from build123d import *

# Parameters (mm, degrees)
SKETCH1_W           = 110.344434204
SKETCH1_H           = 22.05
BOSS_EXTRUDE1_DEPTH = 3
SKETCH3_W           = 10.2
SKETCH3_H           = 3.2
SKETCH3_W_2         = 3.2
SKETCH3_H_2         = 10.372217102
CUT_EXTRUDE1_DEPTH  = 4


with BuildPart() as part:
    # Sketch1 → Boss-Extrude1 (new body)
    with BuildSketch(Plane(origin=(0, 0, 0), x_dir=(1, 0, 0), z_dir=(0, 1, 0))):
        with Locations((0, -55.817990858)):
            Rectangle(SKETCH1_W, SKETCH1_H)
    extrude(amount=-BOSS_EXTRUDE1_DEPTH)

    # Sketch3 → Cut-Extrude1 (cut, through all)
    with BuildSketch(Plane(origin=(0, 0, 0), x_dir=(1, 0, 0), z_dir=(0, 1, 0))):
        with Locations((-40, -46.292990858)):
            Rectangle(SKETCH3_W, SKETCH3_H)
        with Locations((-53.672217102, -61.756882307)):
            Rectangle(SKETCH3_W_2, SKETCH3_H_2)
        with Locations((53.672217102, -65.342990858)):
            Rectangle(SKETCH3_W_2, SKETCH3_H)
        with Locations((-40, -65.342990858)):
            Rectangle(SKETCH3_W, SKETCH3_H)
        with Locations((-20, -46.292990858)):
            Rectangle(SKETCH3_W, SKETCH3_H)
        with Locations((-20, -65.342990858)):
            Rectangle(SKETCH3_W, SKETCH3_H)
        with Locations((0, -46.292990858)):
            Rectangle(SKETCH3_W, SKETCH3_H)
        with Locations((0, -65.342990858)):
            Rectangle(SKETCH3_W, SKETCH3_H)
        with Locations((20, -46.292990858)):
            Rectangle(SKETCH3_W, SKETCH3_H)
        with Locations((20, -65.342990858)):
            Rectangle(SKETCH3_W, SKETCH3_H)
        with Locations((40, -46.292990858)):
            Rectangle(SKETCH3_W, SKETCH3_H)
        with Locations((40, -65.342990858)):
            Rectangle(SKETCH3_W, SKETCH3_H)
        with Locations((-40, -57.242990858)):
            Rectangle(SKETCH3_W, SKETCH3_H)
        with Locations((40, -57.242990858)):
            Rectangle(SKETCH3_W, SKETCH3_H)
        with Locations((-20, -57.242990858)):
            Rectangle(SKETCH3_W, SKETCH3_H)
        with Locations((20, -57.242990858)):
            Rectangle(SKETCH3_W, SKETCH3_H)
        with Locations((0, -57.242990858)):
            Rectangle(SKETCH3_W, SKETCH3_H)
    extrude(amount=-CUT_EXTRUDE1_DEPTH, mode=Mode.SUBTRACT)


solid = part.part
Could you check a few things on this model? Use its own coordinates, in mm. A direction names the side the tool comes from. Give positions to 0.01 mm unless a question says otherwise; leave off trailing zeros. Write each loop counter-clockwise with the first axis right and the second up, starting at its lowest first coordinate (ties: lowest second). Pieces come first, ordered by that corner, then holes. Notation, with made-up numbers: (-32, 66.5) -> (12, 66.5) arc R22 ccw to (12, 99.5) -> close; hole circle Ø7 at (-22.5, 25.5). An arc over 180 degrees is marked (long way). Answer as CSV lines item,"result". Start each with the question number.
(1) Which directions (+Z, -Z, +X, -X, +Y, -Y) give clear straight access to the entire face, cutting with the end or side of a thin tool? Please do faces 1 (the face through (20, -1, 55.643)), 2 (the face through (34.9, -1, 65)), 3 (the face through (-54, -1, 56.571)), 4 (the face through (-10, -1, 66.843)).
(2) If we section it at C-C, the plane y = -1.2: Give the number of separate pieces and of enclosed holes in the cut face, and give its area (3 significant figures).
(3) If we section it at A-A, the plane z = 46.25: Write out the boundary of the cut face in (x, y), and give its area (3 significant figures).
(4) Please list where these lines run through material, in increasing order: line 1 (X direction, y = -1.45, z = 57.75); line 2 (X direction, y = -1.95, z = 55.75); line 3 (Z direction, x = -40.5, y = -0.2).
(5) If we section it at B-B, the plane x = 41.5: Write out the boundary of the cut face in (y, z), and give its area (4 significant figures).
(6) If we mould it in two halves opening along Z, with no side actions, what happens to faces 5 (the face through (10, -1, 66.843)), 6 (the face through (14.9, -1, 46)), 7 (the face through (-14.9, -1, 57)), 8 (the face through (14.9, -1, 57))? For each: +Z half, -Z half, draft (parallel to the pull), parting line (faces both ways), or undercut.
(7) If we section it at D-D, the plane z = 61: Write out the boundary of the cut face in (x, y), and give its area (3 significant figures).
(8) I'm going to push flat-ended pins straight in: pin 1 Ø0.9 at (y, z) = (-2, 65) entering from +X; pin 2 Ø1.5 at (x, y) = (-53, -1.5) entering from +Z; pin 3 Ø0.9 at (y, z) = (-1.5, 65) entering from -X. Where does each tip first touch, or does it pass through?
Answer list:
1,face 1,"+Y, -Y"
1,face 2,"+Z, +Y, -Y"
1,face 3,"+Z, -X, +Y, -Y"
1,face 4,"+Z, +X, -X, +Y, -Y"
2,separate pieces,"1"
2,enclosed holes,"5"
2,area,"1,910 mm^2"
3,outline,"(-55.17, -3) -> (-45.1, -3) -> (-45.1, 0) -> (-55.17, 0) -> close; (-34.9, -3) -> (-25.1, -3) -> (-25.1, 0) -> (-34.9, 0) -> close; (-14.9, -3) -> (-5.1, -3) -> (-5.1, 0) -> (-14.9, 0) -> close; (5.1, -3) -> (14.9, -3) -> (14.9, 0) -> (5.1, 0) -> close; (25.1, -3) -> (34.9, -3) -> (34.9, 0) -> (25.1, 0) -> close; (45.1, -3) -> (55.17, -3) -> (55.17, 0) -> (45.1, 0) -> close"
3,area,"178 mm^2"
4,line 1,"-52.07 to -45.1, -34.9 to -25.1, -14.9 to -5.1, 5.1 to 14.9, 25.1 to 34.9, 45.1 to 55.17"
4,line 2,"-55.17 to -45.1, -34.9 to -25.1, -14.9 to -5.1, 5.1 to 14.9, 25.1 to 34.9, 45.1 to 55.17"
4,line 3,"47.89 to 55.64, 58.84 to 63.74"
5,outline,"(-3, 47.89) -> (0, 47.89) -> (0, 55.64) -> (-3, 55.64) -> close; (-3, 58.84) -> (0, 58.84) -> (0, 63.74) -> (-3, 63.74) -> close"
5,area,"37.95 mm^2"
6,face 5,"+Z half"
6,face 6,"draft"
6,face 7,"undercut"
6,face 8,"undercut"
7,outline,"(-52.07, -3) -> (55.17, -3) -> (55.17, 0) -> (-52.07, 0) -> close"
7,area,"322 mm^2"
8,pin 1,"x = 52.07"
8,pin 2,"z = 56.57"
8,pin 3,"x = -52.07"
